from build123d import *


with BuildPart() as f1:
    # F0 (on Front) → F1 (revolve)
    with BuildSketch(Plane.XZ):
        with BuildLine():
            Line((-33.9725, 114.3), (-35.56, 114.3))
            Line((-35.56, 114.3), (-35.56, 18.050768))
            ThreePointArc((-35.56, 18.050768), (-34.59327, 13.190689), (-31.840256, 9.070512))
            Line((-31.840256, 9.070512), (-27.259872, 4.490128))
            ThreePointArc((-27.259872, 4.490128), (-25.616371, 1.643501), (-25.616371, -1.643501))
            Line((-25.616371, -1.643501), (-35.56, -38.75363))
            Line((-35.56, -38.75363), (-34.026593, -39.164505))
            Line((-34.026593, -39.164505), (-24.082964, -2.054376))
            ThreePointArc((-24.082964, -2.054376), (-24.082964, 2.054376), (-26.13734, 5.61266))
            Line((-26.13734, 5.61266), (-30.717724, 10.193044))
            ThreePointArc((-30.717724, 10.193044), (-33.126611, 13.798199), (-33.9725, 18.050768))
            Line((-33.9725, 18.050768), (-33.9725, 114.3))
        make_face()
    revolve(axis=Axis((0, 0, 37.567748), (0, 0, -1)))


solid = f1.part
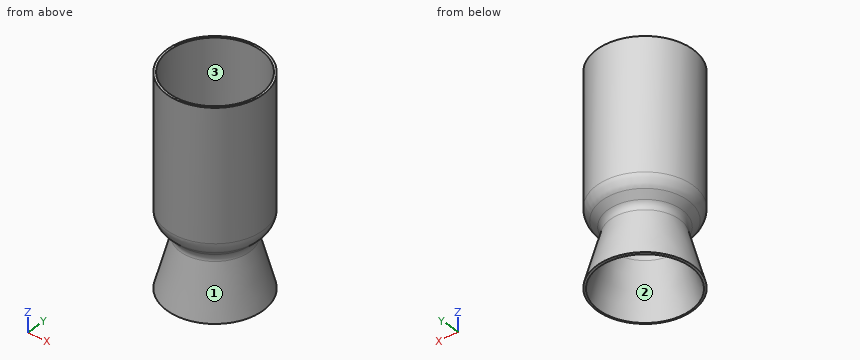
Check sheet for the modelled part. Datum: model origin and axes. Units: mm. Face numbers are marked on the shaded views. Give positions to 0.01 mm unless a question says otherwise; leave off trailing zeros. Order: outer loops, then holes, each group sorted by start corner. A loop starts at its lowest first (then second) coordinate and runs counter-clockwise, first axis right, second up. Notation, with made-up numbers: M 35,88 L 49,88 A34 cw 49,127 Z; hole C -38,7.5 d8. An arc over 180 degrees is marked long. Answer as CSV lines item,"result". Start each with the question number.
Item 1: Gauge pin test, flat ends, axial feed: P1, Ø1.5, axis at x = -6.5, z = 65, coming from the +Y side; P2, Ø1, axis at y = -21, z = 56, coming from the +X side; P3, Ø8, axis at x = -19, y = -16.5, coming from the +Z side. Record the tip position at first contact, or that the pin passes through.
Item 2: Cross-section at C-C on z = 34. Enter the section's corners in (x, y) (1 decimal).
Item 3: Cross-section at D-D on z = -17. Enter the section's corners in (x, y), plus the area to 3 significant figures.
Item 4: Mould release check, pull along X, two halves, no side actions. Record for the marked faces 1, 2 and 3: +X half, -X half, draft (parallel to the pull), parting line (faces both ways), or undercut.
Item 5: Thickness scan on line 1 (X direction, y = 0.5, z = 32.5); line 2 (X direction, y = -6.5, z = -30). Record the ranges inside material, lowest first. Write a range as [from, to].
Established:
1,P1,"stops at y = 35.09"
1,P2,"stops at x = 29.06"
1,P3,"stops at z = 8.64"
2,outline,"C 0,0 d71.1; hole C 0,0 d67.9"
3,outline,"C 0,0 d59.46; hole C 0,0 d56.18"
3,area,"299 mm^2"
4,face 1,"parting line"
4,face 2,"undercut"
4,face 3,"undercut"
5,line 1,"x = [-35.56, -33.97], [33.97, 35.56]"
5,line 2,"x = [-32.57, -30.89], [30.89, 32.57]"
